Design review of the part built by this model. Coordinates are the model's own, in mm. A direction names the side the tool comes from. Coordinates: 2 decimals unless noted, no trailing zeros. One line per item, written item: value.
from build123d import *

# Parameters (mm, degrees)
CHAMFER1_SIZE            = 2
CUT_EXTRUDE1_DEPTH       = 6
CUT_EXTRUDE2_DEPTH       = 42.028953192
FILLET2_R                = 2
CIRPATTERN1_COUNT        = 5
FILLET2_OF_CIRPATTERN1_R = 2
FILLET3_R                = 7.5
FILLET4_R                = 7.5


with BuildPart() as part:
    # Sketch1 → Revolve1 (revolve)
    with BuildSketch(Plane(origin=(0, 0, 0), x_dir=(0, 0, -1), z_dir=(1, 0, 0)), mode=Mode.PRIVATE) as revolve1_sk:
        with BuildLine():
            Line((1, 1.925), (-1, 1.925))
            Line((-1, 1.925), (-6.5, 1.925))
            Line((-6.5, 1.925), (-6.5, 8))
            Line((-6.5, 8), (-1, 8))
            Line((-1, 8), (-1, 26.5))
            Line((-1, 26.5), (-4.201562119, 26.5))
            Line((-4.201562119, 26.5), (-4.201562119, 27.5))
            Line((-4.201562119, 27.5), (-3.201562119, 28.75))
            ThreePointArc((-3.201562119, 28.75), (-1.600781059, 27.5), (0, 28.75))
            Line((0, 28.75), (1, 27.5))
            Line((1, 27.5), (1, 26.5))
            Line((1, 26.5), (1, 1.925))
        make_face()
    revolve(revolve1_sk.sketch.rotate(Axis((0, 0, 0), (0, 0, 1)), 90), axis=Axis((0, 0, 0), (0, 0, 1)))

    # Chamfer1
    chamfer1_edges = [part.edges().sort_by_distance(p)[0] for p in [
        (8, 0, 1),
        (26.5, 0, 1),
        (8, 0, 6.5),
    ]]
    chamfer(chamfer1_edges, length=CHAMFER1_SIZE)

    # Sketch2 → Cut-Extrude1 (cut)
    with BuildSketch(Plane.XY.offset(6.5)):
        Polygon((3.464101615, 6), (-3.464101615, 6), (-6.92820323, 0), (-3.464101615, -6), (3.464101615, -6), (6.92820323, 0), align=None)
    extrude(amount=-CUT_EXTRUDE1_DEPTH, mode=Mode.SUBTRACT)

    # Sketch4 → Cut-Extrude2 (cut, symmetric)
    with BuildSketch(Plane.XY.offset(1)):
        with BuildLine():
            ThreePointArc((-9.025852843, 4.305110968), (-5.877852523, 8.090169944), (-1.305261922, 9.914448614))
            ThreePointArc((-1.305261922, 9.914448614), (-2.56946738, 16.726937639), (-6.08224756, 22.699256918))
            ThreePointArc((-6.08224756, 22.699256918), (-13.812953429, 19.011899368), (-19.708758347, 12.799017323))
            ThreePointArc((-19.708758347, 12.799017323), (-15.114253953, 7.612616689), (-9.025852843, 4.305110968))
        make_face()
        with BuildLine():
            ThreePointArc((-4.080732175, 23.142982196), (0, 23.5), (4.080732175, 23.142982196))
            ThreePointArc((4.080732175, 23.142982196), (1.56147319, 19.047006697), (0, 14.498877126))
            ThreePointArc((0, 14.498877126), (-1.56147319, 19.047006697), (-4.080732175, 23.142982196))
        make_face()
    cut_extrude2 = extrude(amount=CUT_EXTRUDE2_DEPTH, both=True, mode=Mode.SUBTRACT)

    # Fillet2
    fillet2_edges = [part.edges().sort_by_distance(p)[0] for p in [
        (-4.080732175, 23.142982196, 0),
        (4.080732175, 23.142982196, 0),
        (-1.305261922, 9.914448614, 0),
        (-6.08224756, 22.699256918, 0),
        (-9.025852843, 4.305110968, 0),
        (-19.708758347, 12.799017323, 0),
    ]]
    fillet(fillet2_edges, radius=FILLET2_R)

    # CirPattern1: Cut-Extrude2 ×5 about axis
    cirpattern1_axis = Axis((0, 0, 0), (0, 0, 1))
    for i in range(1, CIRPATTERN1_COUNT):
        add(cut_extrude2.rotate(cirpattern1_axis, i * 360 / CIRPATTERN1_COUNT), mode=Mode.SUBTRACT)

    # Fillet2 of CirPattern1
    fillet2_of_cirpattern1_edges = [part.edges().sort_by_distance(p)[0] for p in [
        (-23.271299615, 3.270567873, 0),
        (-20.749268432, 11.032581725, 0),
        (-9.832549076, 1.822355255, 0),
        (-23.467794067, 1.229894972, 0),
        (-6.883545757, -7.25374371, 0),
        (-18.262930094, -14.78902919, 0),
        (-10.30172195, -21.121660088, 0),
        (-16.904485308, -16.324471706, 0),
        (-4.771587603, -8.788171127, 0),
        (-8.421646814, -21.939140023, 0),
        (4.771587603, -8.788171127, 0),
        (8.421646814, -21.939140023, 0),
        (16.904485308, -16.324471706, 0),
        (10.30172195, -21.121660088, 0),
        (6.883545757, -7.25374371, 0),
        (18.262930094, -14.78902919, 0),
        (9.832549076, 1.822355255, 0),
        (23.467794067, 1.229894972, 0),
        (20.749268432, 11.032581725, 0),
        (23.271299615, 3.270567873, 0),
        (9.025852843, 4.305110968, 0),
        (19.708758347, 12.799017323, 0),
        (1.305261922, 9.914448614, 0),
        (6.08224756, 22.699256918, 0),
    ]]
    fillet(fillet2_of_cirpattern1_edges, radius=FILLET2_OF_CIRPATTERN1_R)

    # Fillet3
    # the kernel refuses this fillet: 7.5 mm, written as the material it takes off along each edge
    with BuildSketch(Plane(origin=(0, 0, 4.5), x_dir=(-1, 0, 0), z_dir=(0, 1, 0))) as fillet3_piece_1:
        with BuildLine():
            CenterArc((0.727792874, -3.334394592), FILLET3_R, 14.157365729, 30.842634271)
            Line((6.031093733, 1.968906267), (6.13715975, 2.074972284))
            Line((6.13715975, 2.074972284), (8.106066017, 0.106066017))
            Line((8.106066017, 0.106066017), (8.15, 0))
            ThreePointArc((8.15, 0), (8.15, -0.75), (8.145444143, -1.463312108))
            Line((8.145444143, -1.463312108), (8, -1.5))
        make_face()
    revolve(axis=Axis((0, 0, 4.5), (0, 0, 1)), mode=Mode.SUBTRACT)

    # Fillet4
    fillet4_edges = [part.edges().sort_by_distance(p)[0] for p in [
        (8, 0, 3),
    ]]
    fillet(fillet4_edges, radius=FILLET4_R)


solid = part.part
1. Mouldability with a two-part tool opening along Y and no side actions: class faces 3 (the face through (-23, -14, 4.202)), 4 (the face through (0, -6, 4)), 5 (the face through (5.172, -3.042, 3.542)) as released by +Y, released by -Y, zero draft, split by the parting line, or undercut.
Answer block:
face 3: zero draft
face 4: undercut
face 5: undercut
2. Consider section A-A, the plane x = -18. Give the number of separate pieces and of enclosed holes in the cut face, then the cut area to 3 significant figures.
Answer block:
separate pieces: 4
enclosed holes: 0
area: 53.3 mm^2
3. Wall thickness on line 1 along X through (y, z) = (7, 1.75); line 2 along Z through (x, y) = (13, 23.5); line 3 along X through (y, z) = (-20.5, 2): over which ranges is each line inside the solid? List them lowest first.
Answer block:
line 1: x = -26.6 to -24.26, -6.05 to 6.05, 24.26 to 26.6
line 2: z = -1 to 4.2
line 3: x = -18.4 to -15.17, 15.17 to 18.4
4. Insertion check: pin 1 Ø24.5 at (x, y) = (-3.5, -2) entering from +Z; pin 2 Ø3 at (x, z) = (-1.5, 3.5) entering from -Y; pin 3 Ø6 at (x, y) = (-14.5, 11.5) entering from +Z; pin 4 Ø5 at (x, y) = (0, 0) entering from +Z. Each pin has a flat end and moves straight along its axis. Give the tip position at first contact, or say it passes through.
Answer block:
pin 1: stops at z = 6.5
pin 2: stops at y = -28.75
pin 3: passes through
pin 4: stops at z = 0.5
5. For faces 1 (the face through (-0.1, -23.5, 0)), 2 (the face through (3.45, -26.274, 3.609)), list the 3-axis set-ups (+Z, -Z, +X, -X, +Y, -Y) from which the entire face can be reached by the end or side of a thin tool; tool diameter is ignored.
Answer block:
face 1: +Z, -Z
face 2: +Z
